The listing builds one solid part. Answer for the finished solid, in the listing's coordinates (mm). A direction names the side the tool comes from. Round coordinates to 2 decimals unless told otherwise and drop trailing zeros. Write each loop counter-clockwise with the first axis right and the second up, starting at its lowest first coordinate (ties: lowest second). Pieces come first, ordered by that corner, then holes.
(1) A cutting plane is placed at C-C, the plane z = 2. Give the vertices of the cut face in (x, y) (3 decimals), and give its area (3 significant figures).
(2) A cutting plane is placed at D-D, the plane z = 8.5. Give the vertices of the cut face in (x, y), and give its area (3 significant figures).
(3) Each of these flat-tipped pins is pushed along its axis until it touches: pin 1 Ø21.5 at (x, y) = (0, 0) entering from -Z; pin 2 Ø1 at (x, z) = (-1, 12) entering from +Y; pin 3 Ø3 at (y, z) = (-4.5, 9.5) entering from -X. Where does it stop, or does it pass through?
(4) A cutting plane is placed at B-B, the plane y = 0. Give the vertices of the cut face in (x, z) (3 decimals), and give its area (3 significant figures).
(5) The mould has two halves that part along Y. Classify faces 1 (the face through (-13.76, -19.83, 1.97)), 2 (the face through (0, -13, 0)), 3 (the face through (-2.539, 19.334, 5.493)): +Y half, -Y half, draft (parallel to the pull), parting line (faces both ways), or undercut.
(6) For faces 4 (the face through (-10, 3.2, 10.4)), 5 (the face through (-13.887, -10.648, 10.93)), 6 (the face through (10.6, 20, 2)), determine the directions among +Z, -Z, +X, -X, +Y, -Y from which every point of the face is accessible in a straight line to the end or side of a thin tool.
(7) A cutting plane is placed at A-A, the plane x = 0. Give the vertices of the cut face in (y, z) (3 decimals), and give its area (3 significant figures).
(8) Find the intervals of material crossed by probe 1 along Y at (x, z) = (-12.25, 1.65); probe 2 along Z at (x, y) = (-23.5, 0.5); probe 3 along Z at (x, y) = (13, -13), in increasing order.
from build123d import *

# Parameters (mm, degrees)
SKETCH1_R               = 30
BOSS_EXTRUDE1_DEPTH     = 5
SKETCH2_R               = 19.5
BOSS_EXTRUDE2_DEPTH     = 1
SKETCH3_R               = 17.5
BOSS_EXTRUDE3_DEPTH     = 10
CUT_EXTRUDE1_DEPTH      = 4
CUT_EXTRUDE1_DEPTH_BACK = 4
CUT_EXTRUDE1_START      = -5
SKETCH5_R               = 2.05
SKETCH9_R               = 5.5
CUT_EXTRUDE5_DEPTH      = 4
SKETCH7_R               = 12.025
CUT_EXTRUDE3_DEPTH      = 5
SKETCH8_R               = 10.5
CUT_EXTRUDE4_DEPTH      = 44.829214002


with BuildPart() as part:
    # Sketch1 → Boss-Extrude1 (new body)
    with BuildSketch(Plane.XY):
        Circle(SKETCH1_R)
    extrude(amount=BOSS_EXTRUDE1_DEPTH)

    # Sketch2 → Boss-Extrude2 (add)
    with BuildSketch(Plane.XY.offset(5)):
        Circle(SKETCH2_R)
    extrude(amount=BOSS_EXTRUDE2_DEPTH)

    # Sketch3 → Boss-Extrude3 (add)
    with BuildSketch(Plane.XY.offset(6)):
        Circle(SKETCH3_R)
    extrude(amount=BOSS_EXTRUDE3_DEPTH)

    # Sketch5 → Cut-Extrude1 (cut, two sides: drawn at the far end of the back side and taken through both)
    with BuildSketch(Plane.XY.offset(5).offset(CUT_EXTRUDE1_START - CUT_EXTRUDE1_DEPTH_BACK)):
        with Locations((24.5, 0)):
            Circle(SKETCH5_R)
        with Locations((12.25, -21.217622393)):
            Circle(SKETCH5_R)
        with Locations((-12.25, -21.217622393)):
            Circle(SKETCH5_R)
        with Locations((-24.5, 0)):
            Circle(SKETCH5_R)
        with Locations((-12.25, 21.217622393)):
            Circle(SKETCH5_R)
        with Locations((12.25, 21.217622393)):
            Circle(SKETCH5_R)
    extrude(amount=CUT_EXTRUDE1_DEPTH + CUT_EXTRUDE1_DEPTH_BACK, mode=Mode.SUBTRACT)

    # Sketch9 → Cut-Extrude5 (cut)
    with BuildSketch(Plane(origin=(0, 0, 0), x_dir=(-1, 0, 0), z_dir=(0, 0, -1))):
        Circle(SKETCH9_R)
    extrude(amount=-CUT_EXTRUDE5_DEPTH, mode=Mode.SUBTRACT)

    # Sketch7 → Cut-Extrude3 (cut)
    with BuildSketch(Plane(origin=(0, 0, 0), x_dir=(-1, 0, 0), z_dir=(0, 0, -1))):
        Circle(SKETCH7_R)
    extrude(amount=-CUT_EXTRUDE3_DEPTH, mode=Mode.SUBTRACT)

    # Sketch8 → Cut-Extrude4 (cut, through all)
    with BuildSketch(Plane(origin=(0, 0, 5), x_dir=(-1, 0, 0), z_dir=(0, 0, -1))):
        Circle(SKETCH8_R)
    extrude(amount=-CUT_EXTRUDE4_DEPTH, mode=Mode.SUBTRACT)


solid = part.part
Solutions:
1. outline: circle Ø60 at (0, 0); hole circle Ø4.1 at (-24.5, 0); hole circle Ø4.1 at (-12.25, -21.218); hole circle Ø4.1 at (-12.25, 21.218); hole circle Ø24.05 at (0, 0); hole circle Ø4.1 at (12.25, -21.218); hole circle Ø4.1 at (12.25, 21.218); hole circle Ø4.1 at (24.5, 0)
1. area: 2,290 mm2
2. outline: circle Ø35 at (0, 0); hole circle Ø21 at (0, 0)
2. area: 616 mm2
3. pin 1: stops at z = 5
3. pin 2: stops at y = 17.49
3. pin 3: stops at x = -17.24
4. outline: (-30, 0) - (-26.55, 0) - (-26.55, 4) - (-22.45, 4) - (-22.45, 0) - (-12.025, 0) - (-12.025, 5) - (-10.5, 5) - (-10.5, 16) - (-17.5, 16) - (-17.5, 6) - (-19.5, 6) - (-19.5, 5) - (-30, 5) - close; (10.5, 5) - (12.025, 5) - (12.025, 0) - (22.45, 0) - (22.45, 4) - (26.55, 4) - (26.55, 0) - (30, 0) - (30, 5) - (19.5, 5) - (19.5, 6) - (17.5, 6) - (17.5, 16) - (10.5, 16) - close
4. area: 305 mm2
5. face 1: undercut
5. face 2: draft
5. face 3: parting line
6. face 4: +Z, -Z
6. face 5: +Z
6. face 6: -Z
7. outline: (-30, 0) - (-12.025, 0) - (-12.025, 5) - (-10.5, 5) - (-10.5, 16) - (-17.5, 16) - (-17.5, 6) - (-19.5, 6) - (-19.5, 5) - (-30, 5) - close; (10.5, 5) - (12.025, 5) - (12.025, 0) - (30, 0) - (30, 5) - (19.5, 5) - (19.5, 6) - (17.5, 6) - (17.5, 16) - (10.5, 16) - close
7. area: 338 mm2
8. probe 1: y = -27.38 to -23.27, -19.17 to 19.17, 23.27 to 27.38
8. probe 2: z = 4 to 5
8. probe 3: z = 0 to 6
